Autodesk Inventor part; units mm, degrees
ref_plane "Work Plane1" through (33.575, 0, 0) normal (0, 0, -1) x (1, 0, 0)
ref_plane "YZ Plane" through (0, 0, 0) normal (1, 0, 0) x (0, 1, 0)
ref_plane "XZ Plane" through (0, 0, 0) normal (0, 1, 0) x (-1, 0, 0)
sketch "Skizze1" plane through (0, 0, 0) normal (0, 0, 1) x (1, 0, 0)
  line L0 (0, 0) -> (5, 0)
  line L1 (5, 0) -> (5, 1.5)
  line L2 (5, 1.5) -> (2.65, 1.5)
  line L3 (2.65, 1.5) -> (2.3433, 1.5)
  line L4 (2.3433, 1.5) -> (1.65, 1.5)
  line L5 (1.65, 1.5) -> (0.35, 2.8)
  line L6 (0.35, 2.8) -> (0, 2.8)
  line L7 (0, 2.8) -> (0, 0)
  line L8 (2.65, 1.5) -> (1.65, 1.5) construction
  line L9 (-1, 0) -> (6, 0)
  line L10 (0, 3.36) -> (0, -0.56)
  dimension "d0" = 5
  dimension "d1" = 45
  dimension "d2" = 0.3067
  dimension "d3" = 2.35
  dimension "d4" = 1.65
  dimension "d5" = 3
  dimension "d6" = 3
  dimension "d7" = 5.6
revolve "Körper" add sketch "Skizze1" angle 360 about axis through (0, 0, 0) along (1, 0, 0)
sketch "Skizze2" plane through (0, 0, 0) normal (-1, 0, 0) x (0, 0, 1)
  line L0 (2.8, -0.4) -> (-2.8, -0.4)
  line L1 (-2.8, -0.4) -> (-2.8, 0.4)
  line L2 (-2.8, 0.4) -> (2.8, 0.4)
  line L3 (2.8, 0.4) -> (2.8, -0.4)
  line L4 (0, 0.4) -> (0, -0.4) construction
  line L5 (-2.8, 0) -> (2.8, 0) construction
  line L6 (0, 2.8) -> (0, 0)
  dimension "d15" = 0.8
  dimension "d16" = 5.6
extrude "Loch" cut sketch "Skizze2" against normal blind 0.85
thread "Gewinde"
chamfer "Fase1" distance 0.3067 distance2 0.1534 1 edges at (5, -1.5, 0) measured on face at (5, -0.5112, 0.3316)
ref_plane "Work Plane1" through (33.575, 0, 0) normal (0, 0, -1) x (1, 0, 0)
equation "\"d1\" = 0.5 * SEWI"
equation "\"d2\" = GAL"
equation "\"d4\" = KOH"
equation "\"d5\" = BDM"
equation "\"d6\" = GD"
equation "\"d7\" = KOD"
equation "\"d15\" = SBR"
equation "\"d16\" = KOD"
equation "\"d8\" = STI"
equation "\"d12\" = -0.5 * SPD + 0.5 * GD"
equation "\"d13\" = 0.5 * GAL"
equation "\"NLG\" = 4"
equation "\"GAL\" = 0.61345 * PTC"
equation "\"GEL\" = 1.35"
equation "\"KOH\" = 1.65"
equation "\"KOD\" = 5.6"
equation "\"SEWI\" = 90deg"
equation "\"BDM\" = NND"
equation "\"GD\" = NND"
equation "\"SBR\" = 0.8"
equation "\"STI\" = 0.85"
equation "\"SPD\" = NND - 1.2269 * PTC"
equation "\"GUL\" = 0.61345 * PTC"
equation "\"PTC\" = 0.5"
equation "\"EPV\" = 3.15"
equation "\"THREADDIA\" = 3"
equation "\"TOA\" = 30deg"
equation "\"NND\" = 3"
equation "\"GD1\" = THREADDIA - 1.2269 * PTC"
properties part number "DIN 963 - M3 x 4" material "Edelstahl"
Input: part model. Units: mm. Frame: model coordinates. A direction names the side the tool comes from. Coordinates: 2 decimals unless noted, no trailing zeros. Order: outer loops, then holes, each group sorted by start corner. A loop starts at its lowest first (then second) coordinate and runs counter-clockwise, first axis right, second up.
1. Cut plane D-D, the plane x = 2.8. Return loops of the section in (y, z), plus the area to 3 significant figures.
Checked values:
outline: circle Ø3 at (0, 0)
area: 7.07 mm2
2. Access query for faces 5 (the flat face through (0.85, 0, 0)), 6 (the cylindrical face through (0.2, 2.8, 0.1)). Directions: +Z, -Z, +X, -X, +Y, -Y. A direction counts if a zero-diameter tool reaches every point of the face in a straight line with its end or side. Return the directions, or none.
Checked values:
face 5: +Z, -Z, -X
face 6: +X, -X, +Y
3. Cut plane C-C, the plane x = 0.95. Return loops of the section in (y, z), plus the area to 3 significant figures.
Checked values:
outline: circle Ø4.4 at (0, 0)
area: 15.2 mm2
4. Cut plane A-A, the plane z = 0. Return loops of the section in (x, y).
Checked values:
outline: (0, -2.8) - (0.35, -2.8) - (1.65, -1.5) - (4.85, -1.5) - (5, -1.19) - (5, 1.19) - (4.85, 1.5) - (1.65, 1.5) - (0.35, 2.8) - (0, 2.8) - (0, 0.4) - (0.85, 0.4) - (0.85, -0.4) - (0, -0.4) - close
5. Contact query for flat-ended pins moving along their axis: P1, Ø0.6, axis at y = 0, z = 1, coming from the -X side; P2, Ø1, axis at x = 4, z = -1, coming from the -Y side; P3, Ø2, axis at y = 2, z = 1, coming from the +X side. Output: stop coordinate, or through.
Checked values:
P1: stops at x = 0.85
P2: stops at y = -1.41
P3: stops at x = 4.98
6. Cut plane B-B, the plane y = 0. Return loops of the section in (x, z).
Checked values:
outline: (0.85, -2.3) - (1.65, -1.5) - (4.85, -1.5) - (5, -1.19) - (5, 1.19) - (4.85, 1.5) - (1.65, 1.5) - (0.85, 2.3) - close
7. Draft query along Y for faces 1 (the flat face through (0, 1, 0)), 2 (the cylindrical face through (0.2, -2.8, -0.1)), 3 (the flat face through (0.4, -0.4, 0)), 4 (the cylindrical face through (3.23, -1.5, -0.07)). Return one class per face: +Y half, -Y half, draft (parallel to the pull), parting line (faces both ways), or undercut.
Checked values:
face 1: draft
face 2: -Y half
face 3: undercut
face 4: parting line
8. Ray query, line 1 along X through (y, z) = (0.2, 0.35); line 2 along Z through (x, y) = (3.35, 0.7); line 3 along X through (y, z) = (1.75, 2.1). Return the intervals inside material, ascending.
Checked values:
line 1: x = 0.85 to 5
line 2: z = -1.33 to 1.33
line 3: x = 0 to 0.42
